from build123d import *

# Parameters (mm, degrees)
SKETCH1_R           = 6
SKETCH1_R_2         = 3.2
BOSS_EXTRUDE1_DEPTH = 41.5
SKETCH2_W           = 3
SKETCH2_H           = 5
FILLET1_R           = 5


with BuildPart() as part:
    # Sketch1 → Boss-Extrude1 (new body)
    with BuildSketch(Plane(origin=(0, 0, 0), x_dir=(1, 0, 0), z_dir=(0, 1, 0))):
        with Locations(Location((0, 0, 0), (0, 0, 270))):
            Circle(SKETCH1_R)
        with Locations(Location((0, 0, 0), (0, 0, 270))):
            Circle(SKETCH1_R_2, mode=Mode.SUBTRACT)
    extrude(amount=BOSS_EXTRUDE1_DEPTH)

    # Sketch2 → Revolve1 (revolve)
    with BuildSketch(Plane.XY, mode=Mode.PRIVATE) as revolve1_sk:
        with Locations((7.5, 39)):
            Rectangle(SKETCH2_W, SKETCH2_H)
        with Locations((7.5, 2.5)):
            Rectangle(SKETCH2_W, SKETCH2_H)
    revolve(revolve1_sk.sketch.rotate(Axis((0, 42.288271676, 0), (0, -1, 0)), 90), axis=Axis((0, 42.288271676, 0), (0, -1, 0)))

    # Fillet1
    # the kernel refuses this fillet: 5 mm, written as the material it adds along each edge
    with BuildSketch(Plane(origin=(0, 5, 0), x_dir=(0, 0, 1), z_dir=(1, 0, 0))) as fillet1_piece_1:
        with BuildLine():
            CenterArc((11, -4.582575695), FILLET1_R, 113.578178478, 66.421821522)
            Line((9, 0), (8.96, 0.091651514))
            ThreePointArc((8.96, 0.091651514), (7.5, 0.1), (6, 0.1))
            Line((6, 0.1), (5.9, 0))
            Line((5.9, 0), (5.9, -4.582575695))
            Line((5.9, -4.582575695), (6, -4.582575695))
        make_face()
    revolve(axis=Axis((0, 5, 0), (0, -1, 0)))
    with BuildSketch(Plane(origin=(0, 36.5, 0), x_dir=(0, 0, 1), z_dir=(1, 0, 0))) as fillet1_piece_2:
        with BuildLine():
            CenterArc((11, 4.582575695), FILLET1_R, 180, 66.421821522)
            Line((9, 0), (8.96, -0.091651514))
            ThreePointArc((8.96, -0.091651514), (7.5, -0.1), (6, -0.1))
            Line((6, -0.1), (5.9, 0))
            Line((5.9, 0), (5.9, 4.582575695))
            Line((5.9, 4.582575695), (6, 4.582575695))
        make_face()
    revolve(axis=Axis((0, 36.5, 0), (0, -1, 0)))


solid = part.part
For this review, take the finished solid that the model builds, in its own axes (mm). Round coordinates to 2 decimals unless told otherwise and drop trailing zeros. Write each loop counter-clockwise with the first axis right and the second up, starting at its lowest first coordinate (ties: lowest second). Pieces come first, ordered by that corner, then holes. Notation, with made-up numbers: (84, -19.75) - (135, -19.75) arc R21 cw to (135, 15.25) - close; hole circle Ø8 at (73, 88.5). An arc over 180 degrees is marked (long way). Use a Markdown table: item, result.
Q1. We need section C-C (y = 14). Give the boundary of the cut face in (x, z), plus the area to 3 significant figures.
Derived:
| item | result |
|---|---|
| outline | circle Ø12 at (0, 0); hole circle Ø6.4 at (0, 0) |
| area | 80.9 mm2 |
Q2. We need section B-B (x = 0). Give the boundary of the cut face in (y, z), plus the area to 3 significant figures.
Derived:
| item | result |
|---|---|
| outline | (0, -9) - (5, -9) arc R5 cw to (9.58, -6) - (31.92, -6) arc R5 cw to (36.5, -9) - (41.5, -9) - (41.5, -3.2) - (0, -3.2) - close; (0, 3.2) - (41.5, 3.2) - (41.5, 9) - (36.5, 9) arc R5 cw to (31.92, 6) - (9.58, 6) arc R5 cw to (5, 9) - (0, 9) - close |
| area | 308 mm2 |
Q3. The part is to be moulded in two halves that separate along Y. For faces 1 (the flat face through (4, 41.5, 0)), 2 (the cylindrical face through (1.802, 20.594, 5.723)), 3 (the cylindrical face through (-6.083, 39.035, -6.633)), 4 (the flat face through (4, 0, 0)), say which applies: pulls with the +Y half, pulls with the -Y half, needs draft (parallel to the pull), parting line crosses it, or undercut.
Derived:
| item | result |
|---|---|
| face 1 | pulls with the +Y half |
| face 2 | undercut |
| face 3 | needs draft |
| face 4 | pulls with the -Y half |
Q4. Clearance check with flat-ended pins moving along their axes: pin 1 (10 mm diameter, centred on x = -6.5, y = 6, fed in from +Z); pin 2 (6 mm diameter, centred on y = 34, z = -6, fed in from -X); pin 3 (1.5 mm diameter, centred on x = -4, y = 24, fed in from -Z); pin 4 (6 mm diameter, centred on x = 4, z = -5.5, fed in from -Y). State where each tip first meets the part, or that it passes through.
Derived:
| item | result |
|---|---|
| pin 1 | stops at z = 8.86 |
| pin 2 | stops at x = -7.88 |
| pin 3 | stops at z = -5.04 |
| pin 4 | stops at y = 0 |
Q5. Wall thickness on line 1 along X through (y, z) = (13, 0); line 2 along Y through (x, z) = (-4.25, -7); line 3 along Y through (x, z) = (6.5, -2.5): over which ranges is each line inside the solid? List them lowest first.
Derived:
| item | result |
|---|---|
| line 1 | x = -6 to -3.2, 3.2 to 6 |
| line 2 | y = 0 to 5.45, 36.05 to 41.5 |
| line 3 | y = 0 to 6.63, 34.87 to 41.5 |
Q6. We need section D-D (y = 9). Give the boundary of the cut face in (x, z), plus the area to 3 significant figures.
Derived:
| item | result |
|---|---|
| outline | circle Ø12.07 at (0, 0); hole circle Ø6.4 at (0, 0) |
| area | 82.2 mm2 |
Q7. We need section A-A (z = 0). Give the boundary of the cut face in (x, y), plus the area to 3 significant figures.
Derived:
| item | result |
|---|---|
| outline | (-9, 0) - (-3.2, 0) - (-3.2, 41.5) - (-9, 41.5) - (-9, 36.5) arc R5 cw to (-6, 31.92) - (-6, 9.58) arc R5 cw to (-9, 5) - close; (3.2, 0) - (9, 0) - (9, 5) arc R5 cw to (6, 9.58) - (6, 31.92) arc R5 cw to (9, 36.5) - (9, 41.5) - (3.2, 41.5) - close |
| area | 308 mm2 |
